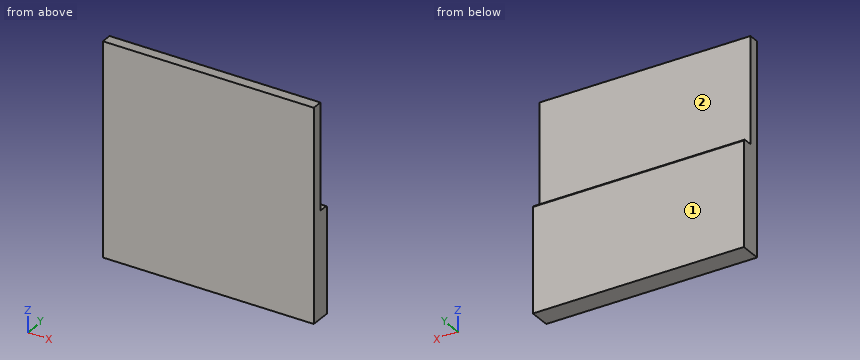
```python
from build123d import *

# Parameters (mm, degrees)
SKETCH1_W           = 2000
SKETCH1_H           = 2000
BOSS_EXTRUDE1_DEPTH = 100
SKETCH2_W           = 2000
SKETCH2_H           = 1000
BOSS_EXTRUDE2_DEPTH = 100
FILLET1_R           = 20


with BuildPart() as part:
    # Sketch1 → Boss-Extrude1 (new body)
    with BuildSketch(Plane(origin=(0, 0, 0), x_dir=(1, 0, 0), z_dir=(0, 1, 0))):
        with Locations((1000, 1000)):
            Rectangle(SKETCH1_W, SKETCH1_H)
    extrude(amount=BOSS_EXTRUDE1_DEPTH)

    # Sketch2 → Boss-Extrude2 (add)
    with BuildSketch(Plane(origin=(0, 100, 0), x_dir=(1, 0, 0), z_dir=(0, 1, 0))):
        with Locations((1000, 1500)):
            Rectangle(SKETCH2_W, SKETCH2_H)
    extrude(amount=BOSS_EXTRUDE2_DEPTH)

    # Fillet1
    fillet1_edges = [part.edges().sort_by_distance(p)[0] for p in [
        (1000, 200, -1000),
    ]]
    fillet(fillet1_edges, radius=FILLET1_R)


solid = part.part
```
Here's how the part is built. I have some questions about the finished solid (model axes, mm). Face numbers are marked on the shaded views. A direction names the side the tool comes from. Round coordinates to 2 decimals unless told otherwise and drop trailing zeros. Write each loop counter-clockwise with the first axis right and the second up, starting at its lowest first coordinate (ties: lowest second). Pieces come first, ordered by that corner, then holes.
Q1. Please list where these lines run through material, in increasing order: probe 1 along Z at (x, y) = (1717, 150.5); probe 2 along Y at (x, z) = (334.5, -119.5).
Q2. If we section it at C-C on y = 133.5: Write out the boundary of the cut face in (x, z), plus the area to 3 significant figures.
Q3. Will this pin go through, and if not, where does the flat tip stop? P1, Ø1.5, axis at x = 1756, y = 161.5, coming from the +Z side.
Q4. Which directions (+Z, -Z, +X, -X, +Y, -Y) give clear straight access to the entire face, cutting with the end or side of a thin tool? Please do the marked faces 1 and 2.
Q5. If we section it at A-A on x = 128: Write out the boundary of the cut face in (y, z).
Q6. If we section it at B-B on z = -724: Write out the boundary of the cut face in (x, y), plus the area to 3 significant figures.
Answer below:
1. probe 1: z = -2000 to -1000
1. probe 2: y = 0 to 100
2. outline: (0, -2000) - (2000, -2000) - (2000, -1000) - (0, -1000) - close
2. area: 2,000,000 mm2
3. P1: stops at z = -1000
4. face 1: +Z, -Z, +X, -X, +Y
4. face 2: +Z, +X, -X, +Y
5. outline: (0, -2000) - (200, -2000) - (200, -1020) arc R20 ccw to (180, -1000) - (100, -1000) - (100, 0) - (0, 0) - close
6. outline: (0, 0) - (2000, 0) - (2000, 100) - (0, 100) - close
6. area: 200,000 mm2
